Could you check a few things on this model? Use its own coordinates, in mm. A direction names the side the tool comes from. Coordinates: 2 decimals unless noted, no trailing zeros. Order: outer loops, then holes, each group sorted by start corner. A loop starts at its lowest first (then second) coordinate and runs counter-clockwise, first axis right, second up. Notation, with made-up numbers: (56.5, 45) - (68.5, 45) arc R26 ccw to (68.5, 73) - close; hole circle Ø6 at (15, -10). An arc over 180 degrees is marked (long way). Answer as a JSON object with one key per item and string values. Group by question number.
(1) Imagine slicing it at D-D, the plane y = 10.5. Write out the boundary of the cut face in (x, z) (3 decimals), and give its area (3 significant figures).
(2) Please list where these lines run through material, in increasing order: probe 1 along Z at (x, y) = (0, -10.75) (3 decimals); probe 2 along X at (y, z) = (-9, 9); probe 3 along Z at (x, y) = (-19, -5).
(3) We'd pull the mould along Y, two halves only. Please class faces 1 (the cylindrical face through (5.265, -7.29, -5.341)), 2 (the flat face through (7, -14.685, 0)), 3 (the flat face through (-30, -12.685, 10)), 4 (the flat face through (-0.2, 14.685, 29.3)): pulls with the +Y half, pulls with the -Y half, needs draft (parallel to the pull), parting line crosses it, or undercut.
(4) Which directions (+Z, -Z, +X, -X, +Y, -Y) give clear straight access to the entire face, cutting with the end or side of a thin tool? Please do faces 5 (the flat face through (-30, 12.685, 10)), 6 (the flat face through (-2, -7, 18)).
(5) Imagine slicing it at C-C, the plane y = -1. Write out the boundary of the cut face in (x, z) (3 decimals), and give its area (3 significant figures).
(6) Will these pins go through, and if not, where does the flat tip stop? P1, Ø1, axis at x = -0.5, z = 10, coming from the +Y side (3 decimals); P2, Ø1, axis at y = -4.5, z = 7.5, coming from the +X side; P3, Ø5, axis at x = 17, z = -6.5, coming from the -Y side; P4, Ø16.5, axis at x = 13.5, y = -7.5, coming from the -Z side.
Autodesk Inventor part; units mm, degrees
ref_plane "YZ Plane" through (0, 0, 0) normal (1, 0, 0) x (0, 1, 0)
ref_plane "XZ Plane" through (0, 0, 0) normal (0, 1, 0) x (-1, 0, 0)
ref_plane "XY Plane" through (0, 0, 0) normal (0, 0, 1) x (1, 0, 0)
sketch "Sketch1" plane through (0, 0, 0) normal (0, 0, 1) x (1, 0, 0)
  line L0 (0, 0) -> (31.095, 0)
  line L1 (31.095, 0) -> (31.095, 14.685)
  line L2 (31.095, 14.685) -> (33.095, 14.685)
  line L3 (33.095, 14.685) -> (33.095, 12.685)
  line L4 (33.095, 12.685) -> (31.095, 12.685)
  line L5 (31.095, 0) -> (31.095, 6.28)
  line L6 (31.095, 6.28) -> (33.095, 6.28)
  line L7 (33.095, 6.28) -> (31.095, 4.3618)
  line L8 (31.095, -14.685) -> (33.095, -14.685)
  line L9 (33.095, -14.685) -> (33.095, -12.685)
  line L10 (33.095, -12.685) -> (31.095, -12.685)
  line L11 (31.095, -6.28) -> (33.095, -6.28)
  line L12 (33.095, -6.28) -> (31.095, -4.3618)
  line L13 (31.095, 14.685) -> (29.095, 14.685)
  line L14 (29.095, 14.685) -> (29.095, -14.685)
  line L15 (29.095, -14.685) -> (31.095, -14.685)
  line L16 (33.095, -6.28) -> (31.095, -4.3618)
  line L17 (31.095, 0) -> (31.095, -4.3618)
  line L18 (31.095, -6.28) -> (31.095, -14.685)
  line L19 (0, -20.559) -> (0, 20.559)
  dimension "d0" = 31.095
  dimension "d1" = 14.685
  dimension "d2" = 2
  dimension "d3" = 2
  dimension "d4" = 6.28
  dimension "d5" = 2
  dimension "d6" = 2
revolve "Revolution1" add sketch "Sketch1" angle 360 about axis through (0, -10, 0) along (0, 1, 0)
sketch "Sketch2" plane through (0, -14.685, 0) normal (0, -1, 0) x (1, 0, 0)
  circle A0 centre (0, 0) radius 29.095
  line L0 (0, 0) -> (-2, 0)
  line L1 (-2, 0) -> (2, 0)
  line L2 (-2, 0) -> (2, 0)
  line L3 (2, 0) -> (2, 29.0262)
  line L4 (-2, 29.0262) -> (-2, 0)
  circle A1 centre (0, 0) radius 7.5
  dimension "d8" = 2
  dimension "d9" = 4
  dimension "d10" = 15
extrude "Extrusion1" add sketch "Sketch2" against normal blind 15 contours L3 A1 L4 A0 | A1 L4 L0 L1 L3 | L3 L1 L0 L4 A1 picked at (-0.2224, 14.6756)
pattern_circular "Circular Pattern1" count 4 over 360 about axis through (0, -14.685, 0) along (0, 1, 0) of "Extrusion1"
sketch "Sketch3" plane through (0, -14.685, 0) normal (0, -1, 0) x (1, 0, 0)
  circle A0 centre (0, 0) radius 2.5
  dimension "d16" = 5
extrude "Extrusion2" cut sketch "Sketch3" against normal blind 15
properties part number "OSV Specific Wheel #2"
Result set:
{
 "1": {"outline": "circle Ø62.19 at (0, 0); hole circle Ø58.19 at (0, 0)", "area": "378 mm^2"},
 "2": {"probe 1": "z = -31.095 to -2.5, 2.5 to 31.095", "probe 2": "x = -29.76 to -27.67, -2 to 2, 27.67 to 29.76", "probe 3": "z = -25.45 to -22.03, -2 to 2, 22.03 to 25.45"},
 "3": {"face 1": "needs draft", "face 2": "pulls with the -Y half", "face 3": "undercut", "face 4": "pulls with the +Y half"},
 "4": {"face 5": "none", "face 6": "+Y, -Y"},
 "5": {"outline": "circle Ø62.19 at (0, 0); hole (-29.026, -2) arc R29.095 ccw to (-2, -29.026) - (-2, -7.228) arc R7.5 cw to (-7.228, -2) - close; hole (-29.026, 2) - (-7.228, 2) arc R7.5 cw to (-2, 7.228) - (-2, 29.026) arc R29.095 ccw to start; hole circle Ø5 at (0, 0); hole (2, -29.026) arc R29.095 ccw to (29.026, -2) - (7.228, -2) arc R7.5 cw to (2, -7.228) - close; hole (2, 7.228) arc R7.5 cw to (7.228, 2) - (29.026, 2) arc R29.095 ccw to (2, 29.026) - close", "area": "882 mm^2"},
 "6": {"P1": "stops at y = 0.315", "P2": "stops at x = 30.88", "P3": "passes through", "P4": "stops at z = -32.66"}
}
